Geometry: final body of the model. Coordinates: model frame, mm. A direction names the side the tool comes from. Round coordinates to 2 decimals unless told otherwise and drop trailing zeros. Write each loop counter-clockwise with the first axis right and the second up, starting at its lowest first coordinate (ties: lowest second). Pieces come first, ordered by that corner, then holes. Notation, with made-up numbers: (49.5, 63.25) -> (88.5, 63.25) arc R29 ccw to (88.5, 101.25) -> close; hole circle Ø5 at (29, 25.25). An arc over 180 degrees is marked (long way). One line per item, written item: value. Start each with the question number.
from build123d import *

# Parameters (mm, degrees)
F1_DEPTH = 3.175
F2_R     = 2.5527
F2_R_2   = 7.9375
F3_DEPTH = 3.176
F4_R     = 9.525
F4_R_2   = 7.9375
F5_DEPTH = 50.8


with BuildPart() as f1:
    # F0 (on Front) → F1 (new body)
    with BuildSketch(Plane.XZ):
        with BuildLine():
            Line((0, 28.575), (0, 0))
            ThreePointArc((0, 0), (12.7, -4.850968), (25.4, 0))
            Line((25.4, 0), (25.4, 28.575))
            ThreePointArc((25.4, 28.575), (12.7, 33.425968), (0, 28.575))
        make_face()
    extrude(amount=-F1_DEPTH)

    # F2 (on face) → F3 (cut, through all)
    with BuildSketch(Plane.XZ):
        with Locations((12.7, 28.575)):
            Circle(F2_R)
        with Locations((12.7, 0)):
            Circle(F2_R)
        with Locations((12.7, 14.2875)):
            Circle(F2_R_2)
        with BuildLine():
            ThreePointArc((25.4, 19.786761), (22.225, 14.2875), (25.4, 8.788239))
            Line((25.4, 8.788239), (25.4, 19.786761))
        make_face()
    extrude(amount=-F3_DEPTH, mode=Mode.SUBTRACT)

    # F4 (on face) → F5 (join)
    with BuildSketch(Plane.XZ):
        with Locations((12.7, 14.2875)):
            Circle(F4_R)
        with Locations((12.7, 14.2875)):
            Circle(F4_R_2, mode=Mode.SUBTRACT)
    extrude(amount=-F5_DEPTH)


solid = f1.part
(1) Section query C-C (x = 16.25). Output: boundary loops of the cut face in (y, z) (3 decimals).
(2) Set-up query: faces 1 (the face through (4, 3.175, 19)), 2 (the face through (14.07, 1.57, 30.73)). Return all of +Z, -Z, +X, -X, +Y, -Y with unobstructed straight access to the full face (end or side cutting, diameter ignored); none if empty.
(3) Section query A-A (x = 12.7). Count the separate pieces of the cut face and the enclosed holes in it, and give its area (3 significant figures).
(4) Pin query (flat end, axial travel): pin 1 (12 mm diameter, centred on x = 9.5, z = 18.5, fed in from -Y); pin 2 (10 mm diameter, centred on x = 19.5, y = 36, fed in from +Z); pin 3 (12 mm diameter, centred on x = 17.5, y = 6, fed in from -Z); pin 4 (5 mm diameter, centred on x = 7.5, y = 39, fed in from -Z). Return the tip coordinate at first contact, or that it passes through.
(5) Line query: probe 1 along Z at (x, y) = (12.7, 1.1) (3 decimals); probe 2 along Z at (x, y) = (12.75, 26.5); probe 3 along Y at (x, z) = (4.75, 3.5) (3 decimals). Output: solid intervals per line, ascending.
(6) Section query B-B (z = 11). Output: boundary loops of the cut face in (x, y) (3 decimals), and give its area (3 significant figures).
Results list:
1. outline: (0, -4.517) -> (3.175, -4.517) -> (3.175, 5.449) -> (50.8, 5.449) -> (50.8, 7.188) -> (0, 7.188) -> close; (0, 21.387) -> (50.8, 21.387) -> (50.8, 23.126) -> (3.175, 23.126) -> (3.175, 33.092) -> (0, 33.092) -> close
2. face 1: +Y
2. face 2: +Y, -Y
3. separate pieces: 4
3. enclosed holes: 0
3. area: 190 mm^2
4. pin 1: stops at y = 0
4. pin 2: stops at z = 23.64
4. pin 3: stops at z = -4.85
4. pin 4: stops at z = 5.15
5. probe 1: z = -4.851 to -2.553, 2.553 to 6.35, 22.225 to 26.022, 31.128 to 33.426
5. probe 2: z = 4.76 to 6.35, 22.22 to 23.81
5. probe 3: y = 0 to 3.175
6. outline: (0, 0) -> (5.475, 0) -> (5.475, 50.8) -> (3.76, 50.8) -> (3.76, 3.175) -> (0, 3.175) -> close; (19.925, 0) -> (23.142, 0) -> (23.142, 3.175) -> (21.64, 3.175) -> (21.64, 50.8) -> (19.925, 50.8) -> close
6. area: 191 mm^2
